```python
from build123d import *

# Parameters (mm, degrees)
F0_R     = 44.45
F1_DEPTH = 6.35
F2_R     = 9.525
F3_DEPTH = 3.175
F4_R     = 1.2827
F5_DEPTH = 25.4


with BuildPart() as f1:
    # F0 (on Top) → F1 (new body)
    with BuildSketch(Plane.XY):
        Circle(F0_R)
    extrude(amount=F1_DEPTH)

    # F2 (on face) → F3 (cut)
    with BuildSketch(Plane.XY.offset(6.35)):
        with Locations((-28.575, 0)):
            Circle(F2_R)
        with Locations((-14.2875, 24.746676)):
            Circle(F2_R)
        with Locations((14.2875, 24.746676)):
            Circle(F2_R)
        with Locations((28.575, 0)):
            Circle(F2_R)
        Circle(F2_R)
        with Locations((14.2875, -24.746676)):
            Circle(F2_R)
        with Locations((-14.2875, -24.746676)):
            Circle(F2_R)
    extrude(amount=-F3_DEPTH, mode=Mode.SUBTRACT)

    # F4 (on face) → F5 (cut)
    with BuildSketch(Plane.XY.offset(6.35)):
        with Locations((28.575, 0)):
            Circle(F4_R)
        Circle(F4_R)
        with Locations((-14.2875, 24.746676)):
            Circle(F4_R)
        with Locations((14.2875, 24.746676)):
            Circle(F4_R)
        with Locations((-28.575, 0)):
            Circle(F4_R)
        with Locations((-14.2875, -24.746676)):
            Circle(F4_R)
        with Locations((14.2875, -24.746676)):
            Circle(F4_R)
    extrude(amount=-F5_DEPTH, mode=Mode.SUBTRACT)


solid = f1.part
```
Here's how the part is built. I have some questions about the finished solid (model axes, mm). A direction names the side the tool comes from. Round coordinates to 2 decimals unless told otherwise and drop trailing zeros. Loops run counter-clockwise (first coordinate to the right, second up) from the corner with the lowest first, then second, coordinate; pieces in that order, holes last.
1. Suppose I cut it at B-B, the plane x = 0. Please give me the cut outline in (y, z) (3 decimals), and give its area (3 significant figures).
Answers:
outline: (-44.45, 0) - (-1.283, 0) - (-1.283, 3.175) - (-9.525, 3.175) - (-9.525, 6.35) - (-44.45, 6.35) - close; (1.283, 0) - (44.45, 0) - (44.45, 6.35) - (9.525, 6.35) - (9.525, 3.175) - (1.283, 3.175) - close
area: 496 mm2
2. Suppose I cut it at A-A, the plane y = 0. Please give me the cut outline in (x, z) (3 decimals), and give its area (3 significant figures).
Answers:
outline: (-44.45, 0) - (-29.858, 0) - (-29.858, 3.175) - (-38.1, 3.175) - (-38.1, 6.35) - (-44.45, 6.35) - close; (-27.292, 0) - (-1.283, 0) - (-1.283, 3.175) - (-9.525, 3.175) - (-9.525, 6.35) - (-19.05, 6.35) - (-19.05, 3.175) - (-27.292, 3.175) - close; (1.283, 0) - (27.292, 0) - (27.292, 3.175) - (19.05, 3.175) - (19.05, 6.35) - (9.525, 6.35) - (9.525, 3.175) - (1.283, 3.175) - close; (29.858, 0) - (44.45, 0) - (44.45, 6.35) - (38.1, 6.35) - (38.1, 3.175) - (29.858, 3.175) - close
area: 359 mm2
3. If I drill on probe 1 along Y at (x, z) = (-6, 4.75); probe 2 along Y at (x, z) = (22.5, 5.25); probe 3 along X at (y, z) = (19, 5.75), over which ranges is the centre line in solid material (lowest first)?
Answers:
probe 1: y = -44.04 to -29.44, -20.05 to -7.4, 7.4 to 20.05, 29.44 to 44.04
probe 2: y = -38.33 to -29.57, -19.92 to -7.34, 7.34 to 19.92, 29.57 to 38.33
probe 3: x = -40.18 to -21.88, -6.69 to 6.69, 21.88 to 40.18
4. Will these pins go through, and if not, where does the flat tip stop? pin 1 (2 mm diameter, centred on x = 14.29, y = 24.75, fed in from +Z); pin 2 (4 mm diameter, centred on x = 14.29, y = -24.75, fed in from +Z) (3 decimals); pin 3 (1 mm diameter, centred on x = 34, z = 1, fed in from -Y); pin 4 (1 mm diameter, centred on y = 26.5, z = 4, fed in from +X).
Answers:
pin 1: passes through
pin 2: stops at z = 3.175
pin 3: stops at y = -29.22
pin 4: stops at x = 36.05
5. Suppose I cut it at D-D, the plane x = -11. Please give me the cut outline in (y, z) (3 decimals), and give its area (3 significant figures).
Answers:
outline: (-43.067, 0) - (43.067, 0) - (43.067, 6.35) - (33.686, 6.35) - (33.686, 3.175) - (15.807, 3.175) - (15.807, 6.35) - (-15.807, 6.35) - (-15.807, 3.175) - (-33.686, 3.175) - (-33.686, 6.35) - (-43.067, 6.35) - close
area: 433 mm2
6. For faces 5 (the face through (-1, 11, 6.35)), 6 (the face through (-12, 25, 3.175)), which set-ups out of +Z, -Z, +X, -X, +Y, -Y let a thin tool reach every point of the face, with its end or its side?
Answers:
face 5: +Z, +X, -X, +Y, -Y
face 6: +Z
7. Thinking about a two-plate mould opening in X: for faces 1 (the face through (-1, -9, 0)), 2 (the face through (-14.454, -23.475, 1.61)), 3 (the face through (42.397, 13.352, 3.131)), 4 (the face through (13.34, 25.61, 1.61)), which applies, released by +X, released by -X, zero draft, split by the parting line, or undercut?
Answers:
face 1: zero draft
face 2: undercut
face 3: split by the parting line
face 4: undercut
8. Suppose I cut it at C-C, the plane z = 1. Give the number of separate pieces and of enclosed holes in the cut face, and give its area (3 significant figures).
Answers:
separate pieces: 1
enclosed holes: 7
area: 6,170 mm2
